```python
from build123d import *

# Parameters (mm, degrees)
BOSS_EXTRUDE1_DEPTH = 1.5
SKETCH3_R           = 2.05
CUT_EXTRUDE1_DEPTH  = 26.646259474
SKETCH4_R           = 4.075
CUT_EXTRUDE2_DEPTH  = 3


with BuildPart() as part:
    # Sketch2 → Boss-Extrude1 (new, symmetric)
    with BuildSketch(Plane.XY):
        with BuildLine():
            Line((-13.425, 10), (13.425, 10))
            ThreePointArc((13.425, 10), (23.425, 0), (13.425, -10))
            Line((13.425, -10), (-13.425, -10))
            ThreePointArc((-13.425, -10), (-23.425, 0), (-13.425, 10))
        make_face()
    extrude(amount=BOSS_EXTRUDE1_DEPTH, both=True)

    # Sketch3 → Cut-Extrude1 (cut, through all)
    with BuildSketch(Plane.XY.offset(1.5)):
        with Locations((4.425, 0)):
            Circle(SKETCH3_R)
        with Locations((17.425, 0)):
            Circle(SKETCH3_R)
    extrude(amount=-CUT_EXTRUDE1_DEPTH, mode=Mode.SUBTRACT)

    # Sketch4 → Cut-Extrude2 (cut)
    with BuildSketch(Plane.XY.offset(1.5)):
        with Locations((-11.75, 0.925)):
            Circle(SKETCH4_R)
    extrude(amount=-CUT_EXTRUDE2_DEPTH, mode=Mode.SUBTRACT)


solid = part.part
```
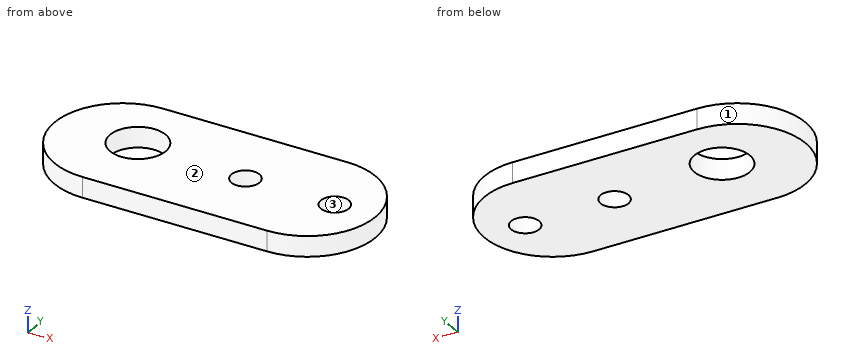
The listing builds one solid part. Answer for the finished solid, in the listing's coordinates (mm). Face numbers are marked on the shaded views. Coordinates: 2 decimals unless noted, no trailing zeros. Loops run counter-clockwise (first coordinate to the right, second up) from the corner with the lowest first, then second, coordinate; pieces in that order, holes last. Notation, with made-up numbers: M 45,-4 L 84,-4 A25 ccw 84,23 Z; hole C 19,9.5 d3. An arc over 180 degrees is marked long. Answer as a JSON object with one key per item and string values. Group by question number.
Item 1: Section A-A (x = -11.75) is taken. Write down the section's boundary in (y, z), and give its area (4 significant figures).
Item 2: Determine the mould class of the marked faces 1, 2 and 3 for opening direction Y: +Y half, -Y half, draft (parallel to the pull), parting line (faces both ways), or undercut.
Item 3: Consider L1, parallel to Y at x = -11.75, z = -0.7; L2, parallel to X at y = -1, z = -0.55; L3, parallel to X at y = -1.5, z = -0.85. Determine where each line is inside the solid, lowest interval first.
Item 4: This flat-tipped pin is pushed along its axis until it touches: P1, Ø3.5, axis at x = 4.425, y = 0, coming from the +Z side. Where does it stop, or does it pass through?
Item 5: Section D-D (y = 3) is taken. Write down the section's boundary in (x, z).
Item 6: Section B-B (y = 0) is taken. Write down the section's boundary in (x, z) (3 decimals), and give its area (3 significant figures).
Item 7: Section C-C (z = -0.45) is taken. Write down the section's boundary in (x, y) (3 decimals).
Solved:
{
 "1": {"outline": "M -10,-1.5 L -3.15,-1.5 L -3.15,1.5 L -10,1.5 Z; M 5,-1.5 L 10,-1.5 L 10,1.5 L 5,1.5 Z", "area": "35.55 mm2"},
 "2": {"face 1": "parting line", "face 2": "draft", "face 3": "undercut"},
 "3": {"L1": "y = -10 to -3.15, 5 to 10", "L2": "x = -23.37 to -15.34, -8.16 to 2.64, 6.21 to 15.64, 19.21 to 23.37", "L3": "x = -23.31 to -15.02, -8.48 to 3.03, 5.82 to 16.03, 18.82 to 23.31"},
 "4": {"P1": "passes through"},
 "5": {"outline": "M -22.96,-1.5 L -15.26,-1.5 L -15.26,1.5 L -22.96,1.5 Z; M -8.24,-1.5 L 22.96,-1.5 L 22.96,1.5 L -8.24,1.5 Z"},
 "6": {"outline": "M -23.425,-1.5 L -15.719,-1.5 L -15.719,1.5 L -23.425,1.5 Z; M -7.781,-1.5 L 2.375,-1.5 L 2.375,1.5 L -7.781,1.5 Z; M 6.475,-1.5 L 15.375,-1.5 L 15.375,1.5 L 6.475,1.5 Z; M 19.475,-1.5 L 23.425,-1.5 L 23.425,1.5 L 19.475,1.5 Z", "area": "92.1 mm2"},
 "7": {"outline": "M -13.425,-10 L 13.425,-10 A10 ccw 13.425,10 L -13.425,10 A10 ccw Z; hole C -11.75,0.925 d8.15; hole C 4.425,0 d4.1; hole C 17.425,0 d4.1"}
}
